from build123d import *

# Parameters (mm, degrees)
EXTRUDE17_DEPTH = 1.6129
EXTRUDE19_START = -4.2291
SKETCH19_R      = 3.6195
EXTRUDE19_DEPTH = 4.2291
SKETCH20_R      = 0.46355
SKETCH20_R_2    = 1.27
EXTRUDE20_DEPTH = 18.050548166
SKETCH21_R      = 2.44475
EXTRUDE21_DEPTH = 1.1557
SKETCH22_R      = 2.286
EXTRUDE22_DEPTH = 2.3368
SKETCH23_R      = 2.159
EXTRUDE23_DEPTH = 0.2032
SKETCH24_R      = 1.651
EXTRUDE24_DEPTH = 0.762
EXTRUDE25_DEPTH = 0.508
FILLET1_R       = 0.508


with BuildPart() as part:
    # Sketch18 → Extrude17 (new body)
    with BuildSketch(Plane(origin=(0, 0, 0), x_dir=(1, 0, 0), z_dir=(0, 1, 0))):
        with BuildLine():
            Line((-14.34305969, 1.923991942), (-2.13741415, 2.921))
            ThreePointArc((-2.13741415, 2.921), (0, 3.6195), (2.13741415, 2.921))
            Line((2.13741415, 2.921), (14.34305969, 1.923991942))
            ThreePointArc((14.34305969, 1.923991942), (16.1163, 0), (14.34305969, -1.923991942))
            Line((14.34305969, -1.923991942), (2.13741415, -2.921))
            ThreePointArc((2.13741415, -2.921), (0, -3.6195), (-2.13741415, -2.921))
            Line((-2.13741415, -2.921), (-14.34305969, -1.923991942))
            ThreePointArc((-14.34305969, -1.923991942), (-16.1163, 0), (-14.34305969, 1.923991942))
        make_face()
    extrude(amount=EXTRUDE17_DEPTH)

    # Sketch19 → Extrude19 (add)
    with BuildSketch(Plane(origin=(0, 1.6129, 0), x_dir=(1, 0, 0), z_dir=(0, 1, 0)).offset(EXTRUDE19_START)):
        with Locations(Location((0, 0, 0), (0, 0, 126.194447475))):
            Circle(SKETCH19_R)
    extrude(amount=EXTRUDE19_DEPTH)

    # Sketch20 → Extrude20 (cut, through all)
    with BuildSketch(Plane(origin=(0, 1.6129, 0), x_dir=(1, 0, 0), z_dir=(0, 1, 0))):
        with Locations(Location((-14.1859, 0, 0), (0, 0, 270))):
            Circle(SKETCH20_R)
        with Locations(Location((0, 0, 0), (0, 0, 270))):
            Circle(SKETCH20_R_2)
        with Locations(Location((-4.6609, 0, 0), (0, 0, 270))):
            Circle(SKETCH20_R)
        with Locations(Location((-6.5659, 0, 0), (0, 0, 270))):
            Circle(SKETCH20_R)
        with Locations(Location((-8.4709, 0, 0), (0, 0, 270))):
            Circle(SKETCH20_R)
        with Locations(Location((-10.3759, 0, 0), (0, 0, 270))):
            Circle(SKETCH20_R)
        with Locations(Location((-12.2809, 0, 0), (0, 0, 270))):
            Circle(SKETCH20_R)
    extrude20 = extrude(amount=-EXTRUDE20_DEPTH, mode=Mode.SUBTRACT)

    # Sketch21 → Extrude21 (cut)
    with BuildSketch(Plane(origin=(0, 1.6129, 0), x_dir=(1, 0, 0), z_dir=(0, 1, 0))):
        with Locations(Location((0, 0, 0), (0, 0, 270))):
            Circle(SKETCH21_R)
    extrude(amount=-EXTRUDE21_DEPTH, mode=Mode.SUBTRACT)

    # Sketch22 → Extrude22 (cut)
    with BuildSketch(Plane.XZ.offset(2.6162)):
        with Locations(Location((0, 0, 0), (0, 0, 270))):
            Circle(SKETCH22_R)
    extrude(amount=-EXTRUDE22_DEPTH, mode=Mode.SUBTRACT)



with BuildPart() as body_2:
    # Sketch23 → Extrude23 (new body)
    with BuildSketch(Plane(origin=(0, 0.4572, 0), x_dir=(1, 0, 0), z_dir=(0, 1, 0))):
        with Locations(Location((0, 0, 0), (0, 0, 270))):
            Circle(SKETCH23_R)
    extrude(amount=EXTRUDE23_DEPTH)


with BuildPart() as part_1:
    add(part.part)

    add(body_2.part)  # Extrude24 merges body 2
    # Sketch24 → Extrude24 (add)
    with BuildSketch(Plane(origin=(0, 0.6604, 0), x_dir=(1, 0, 0), z_dir=(0, 1, 0))):
        with Locations(Location((0, 0, 0), (0, 0, 90))):
            Circle(SKETCH24_R)
    extrude(amount=EXTRUDE24_DEPTH)

    # Sketch25 → Extrude25 (cut)
    with BuildSketch(Plane(origin=(0, 1.4224, 0), x_dir=(1, 0, 0), z_dir=(0, 1, 0))):
        Polygon((0.254, -1.016), (-0.254, -1.016), (-0.254, -0.254), (-1.016, -0.254), (-1.016, 0.254), (-0.254, 0.254), (-0.254, 1.016), (0.254, 1.016), (0.254, 0.254), (1.016, 0.254), (1.016, -0.254), (0.254, -0.254), align=None)
    extrude(amount=-EXTRUDE25_DEPTH, mode=Mode.SUBTRACT)

    # Fillet1
    fillet1_edges = [part_1.edges().sort_by_distance(p)[0] for p in [
        (0, 1.4224, 1.651),
    ]]
    fillet(fillet1_edges, radius=FILLET1_R)

    # Mirror1: Extrude20 across plane
    add(extrude20.mirror(Plane(origin=(0, 0, 0), x_dir=(0, 0, 1), z_dir=(1, 0, 0))), mode=Mode.SUBTRACT)


solid = part_1.part
Geometry check sheet. Reference: the model listing, model coordinates, mm. A direction names the side the tool comes from. Round coordinates to 2 decimals unless told otherwise and drop trailing zeros. Order: outer loops, then holes, each group sorted by start corner. A loop starts at its lowest first (then second) coordinate and runs counter-clockwise, first axis right, second up. Notation, with made-up numbers: (84.5, -5) - (138.5, -5) arc R20 cw to (138.5, 28) - close; hole circle Ø7 at (6.5, 57.5). An arc over 180 degrees is marked (long way). One line per question, with ' | ' between items. Start each with the question number.
(1) Depth check by flat-ended pin: pin 1 Ø3.5 at (x, z) = (0, 0) entering from +Y; pin 2 Ø4 at (x, z) = (0, 0) entering from -Y; pin 3 Ø3 at (x, z) = (-7, 0) entering from -Y. Enter the tip coordinate at first touch or a pass-through.
(2) Release check for a two-part mould opening along X. For faces 4 (the flat face through (-9, 0, 1)), 5 (the cylindrical face through (-14.64, 0.82, -0.1)), 6 (the cylindrical face through (16.116, 0.795, -0.04)) record: released by +X, released by -X, zero draft, split by the parting line, or undercut.
(3) Sectioned sample at A-A on x = 0. Record the cut outline in (y, z), and give its area (3 significant figures).
(4) Thickness scan on L1, parallel to Y at x = 4, z = -1; L2, parallel to X at y = -1.9, z = -1; L3, parallel to X at y = -1.35, z = -0.5. Record the ranges inside material, lowest first. Write a range as [from, to].
(5) Sectioned sample at B-B on z = 0. Count the separate pieces of the cut face and the enclosed holes in it, and give its area (3 significant figures).
(6) Access from +Z, -Z, +X, -X, +Y, -Y to the whole of each face (thin tool, end or side, straight path). Record for faces 1 (the cylindrical face through (-2.387, 1.043, -0.53)), 2 (the cylindrical face through (14.64, 0.82, -0.1)), 3 (the flat face through (-1.5, -0.279, 0)).
(7) Sectioned sample at C-C on y = -1.4. Record the cut outline in (x, z).
Conclusion:
1) pin 1: stops at y = 1.41 | pin 2: stops at y = -0.28 | pin 3: stops at y = 0
2) face 4: zero draft | face 5: undercut | face 6: released by +X
3) outline: (-2.62, -3.62) - (1.61, -3.62) - (1.61, -2.44) - (0.46, -2.44) - (0.46, -2.16) - (0.66, -2.16) - (0.66, -1.65) - (0.91, -1.65) arc R0.51 ccw to (1.41, -1.27) - (-0.28, -1.27) - (-0.28, -2.29) - (-2.62, -2.29) - close; (-2.62, 2.29) - (-0.28, 2.29) - (-0.28, 1.27) - (1.41, 1.27) arc R0.51 ccw to (0.91, 1.65) - (0.66, 1.65) - (0.66, 2.16) - (0.46, 2.16) - (0.46, 2.44) - (1.61, 2.44) - (1.61, 3.62) - (-2.62, 3.62) - close | area: 13.2 mm2
4) L1: y = [0, 1.61] | L2: x = [-3.48, -2.06], [2.06, 3.48] | L3: x = [-3.58, -2.23], [2.23, 3.58]
5) separate pieces: 14 | enclosed holes: 0 | area: 35.6 mm2
6) face 1: +Y | face 2: +Y, -Y | face 3: -Y
7) outline: circle Ø7.24 at (0, 0); hole circle Ø4.57 at (0, 0)
